Read the model definition and answer for the solid it produces. Units are mm, in the model's axes. Face numbers are marked on the shaded views. A direction names the side the tool comes from. Coordinates: 2 decimals unless noted, no trailing zeros. Order: outer loops, then holes, each group sorted by start corner. A loop starts at its lowest first (then second) coordinate and runs counter-clockwise, first axis right, second up. Notation, with made-up numbers: (7, 17) -> (37, 17) arc R19 ccw to (37, 21) -> close; hole circle Ø7 at (71.25, 35). An arc over 180 degrees is marked (long way). Answer as a JSON object with one key per item and string values. Group by question number.
1) Section A-A on y = 0 is taken. Determine the outline of the cut face in (x, z) (3 decimals).
2) Determine the mould class of the marked faces 4, 5, 6 and 7 for opening direction Y: released by +Y, released by -Y, zero draft, split by the parting line, or undercut.
3) Given pin 1 (8 mm diameter, centred on x = -3, z = 5, fed in from -Y); pin 2 (1 mm diameter, centred on y = -1.5, z = -3, fed in from +X); pin 3 (1.3 mm diameter, centred on y = 0, z = 5, fed in from -X), each flat-ended and moving along its own axis, determine where each tip first touches the part or whether it passes through.
4) A tool of negligible diameter and unlimited length cuts with its end or side. For the marked faces 1, 2 and 3, from which of +Z, -Z, +X, -X, +Y, -Y can it reach the whole face along a straight path? Write none if from no direction.
5) Consider L1, parallel to Y at x = 0, z = -0.75; L2, parallel to Y at x = 0, z = 7 (3 decimals); L3, parallel to Z at x = 5.5, y = -7. Determine where each line is inside the solid, lowest interval first.
6) Section C-C on z = -2 is taken. Determine the outline of the cut face in (x, y).
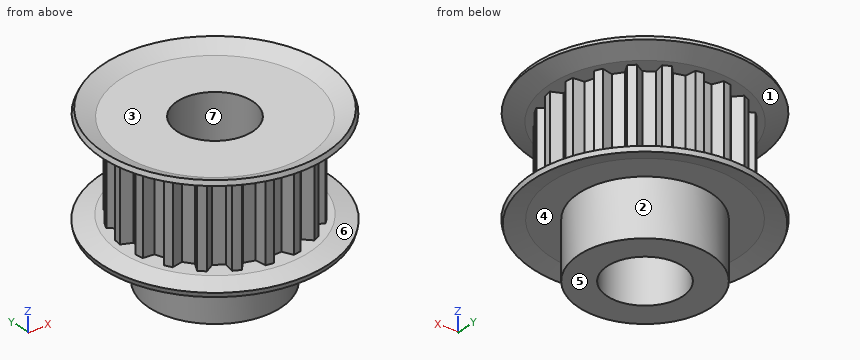
from build123d import *

# Parameters (mm, degrees)
ESQUISSE1_R                  = 9.345000000000002
EXTRUSION1_DEPTH             = 10
EXTRUSION2_DEPTH             = 17.572810564294763
R_P_TITION_CIRCULAIRE1_COUNT = 20
ESQUISSE4_R                  = 4
EXTRUSION3_DEPTH             = 17.50568653417299


with BuildPart() as part:
    # Esquisse1 → Extrusion1 (new body)
    with BuildSketch(Plane.XY):
        Circle(ESQUISSE1_R)
    extrude(amount=EXTRUSION1_DEPTH)

    # Esquisse2 → Extrusion2 (cut, through all)
    with BuildSketch(Plane.XY.offset(10)):
        Polygon((-0.5685000000000011, 8.245), (0.5684999999999989, 8.245), (1.2888044910509866, 9.789697965932955), (-1.2888044910509753, 9.789697965932955), align=None)
    extrusion2 = extrude(amount=-EXTRUSION2_DEPTH, mode=Mode.SUBTRACT)

    # Répétition circulaire1: Extrusion2 ×20 about axis
    r_p_tition_circulaire1_axis = Axis((3e-17, -4.2e-16, 0), (0, 0, 1))
    for i in range(1, R_P_TITION_CIRCULAIRE1_COUNT):
        add(extrusion2.rotate(r_p_tition_circulaire1_axis, i * 360 / R_P_TITION_CIRCULAIRE1_COUNT), mode=Mode.SUBTRACT)

    # Esquisse4 → Extrusion3 (cut, through all)
    with BuildSketch(Plane.XY.offset(10)):
        Circle(ESQUISSE4_R)
    extrude(amount=-EXTRUSION3_DEPTH, mode=Mode.SUBTRACT)

    # Esquisse5 → Révolution1 (revolve)
    with BuildSketch(Plane(origin=(0, 0, 0), x_dir=(0, 0, -1), z_dir=(1, 0, 0)), mode=Mode.PRIVATE) as r_volution1_sk:
        Polygon((-10, 8), (-10, 9.969000000000001), (-10.812476697134908, 11.762555858236022), (-10.357028282143537, 11.96887294740182), (-9.479176274054629, 10.031), (-9.479176274054645, 8), align=None)
        Polygon((0, 8), (-5.9e-16, 9.969000000000001), (0.48091741384473186, 11.878366240683253), (-0.00393942736482848, 12.00048848899324), (-0.5, 10.031), (-0.4999999999999998, 8), align=None)
        Polygon((0, 7), (6, 6.999999999999999), (6.000000000000001, 4), (4.6e-16, 4), align=None)
    revolve(r_volution1_sk.sketch.rotate(Axis((0, 0, -0.6503339320090771), (0, 0, 1)), 90), axis=Axis((0, 0, -0.6503339320090771), (0, 0, 1)))


solid = part.part
Worked answers:
{
 "1": {"outline": "(-12, 0.004) -> (-11.878, -0.481) -> (-9.969, 0) -> (-7, 0) -> (-7, -6) -> (-4, -6) -> (-4, 10) -> (-9.969, 10) -> (-11.763, 10.812) -> (-11.969, 10.357) -> (-10.031, 9.479) -> (-8.245, 9.479) -> (-8.245, 0.5) -> (-10.031, 0.5) -> close; (4, -6) -> (7, -6) -> (7, 0) -> (9.969, 0) -> (11.878, -0.481) -> (12, 0.004) -> (10.031, 0.5) -> (8.245, 0.5) -> (8.245, 9.479) -> (10.031, 9.479) -> (11.969, 10.357) -> (11.763, 10.812) -> (9.969, 10) -> (4, 10) -> close"},
 "2": {"face 4": "undercut", "face 5": "zero draft", "face 6": "split by the parting line", "face 7": "undercut"},
 "3": {"pin 1": "stops at y = -9.29", "pin 2": "stops at x = 6.93", "pin 3": "stops at x = -8.42"},
 "4": {"face 1": "none", "face 2": "-Z", "face 3": "+Z"},
 "5": {"L1": "y = -7 to -4, 4 to 7", "L2": "y = -8.245 to -4, 4 to 8.245", "L3": "z = 0 to 0.5, 9.48 to 10"},
 "6": {"outline": "circle Ø14 at (0, 0); hole circle Ø8 at (0, 0)"}
}
